For this review, take the finished solid that the model builds, in its own axes (mm). A direction names the side the tool comes from. Coordinates: 2 decimals unless noted, no trailing zeros. Loops run counter-clockwise (first coordinate to the right, second up) from the corner with the lowest first, then second, coordinate; pieces in that order, holes last. Notation, with made-up numbers: (-5.75, 58) - (52.25, 58) arc R22 ccw to (52.25, 88) - close; hole circle Ø5 at (-26.5, 85.25). An arc over 180 degrees is marked (long way). One line per item, written item: value. Start each with the question number.
1. Take a section at D-D, the plane y = -0.3. Count the separate pieces of the cut face and the enclosed holes in it, and give its area (3 significant figures).
2. The part is to be moulded in two halves that separate along Z. For faces 1 (the face through (-1.356, 1, -6)), 2 (the face through (0.739, 0.144, -15.866)), 3 (the face through (0.67, 0.27, -6.81)), say which applies: released by +Z, released by -Z, zero draft, split by the parting line, or undercut.
3. To check wall thickness, follow line 1 (Z direction, x = 1, y = 0.2); line 2 (X direction, y = 1.2, z = -15); line 3 (Z direction, x = 0.6, y = -0.75). State the ranges of each line that lie inside material, in increasing order. Write a range as from..to.
4. Take a section at C-C, the plane x = -1.05. State the section outline as (y, z) points.
5. Take a section at A-A, the plane x = 0.55. State the section outline as (y, z) points, and give its area (3 significant figures).
6. Insertion check: pin 1 (1.5 mm diameter, centred on x = -0.5, y = -0.5, fed in from +Z); pin 2 (1.5 mm diameter, centred on x = 0.5, z = -13.5, fed in from -Y) (3 decimals). Each pin has a flat end and moves straight along its axis. Give the tip position at first contact, or say it passes through.
7. For faces 4 (the face through (0.069, -1, -7)), 5 (the face through (0.739, 0.144, -17.695)), list the 3-axis set-ups (+Z, -Z, +X, -X, +Y, -Y) from which the entire face can be reached by the end or side of a thin tool; tool diameter is ignored.
8. Take a section at B-B, the plane z = -11.5. State the section outline as (x, y) points.
```python
from build123d import *

# Parameters (mm, degrees)
BOSS_EXTRUDE1_DEPTH = 2.9972
CUT_EXTRUDE1_DEPTH  = 1.524
SKETCH6_R           = 1.1176
CUT_EXTRUDE3_DEPTH  = 29.630171982
CUT_EXTRUDE4_DEPTH  = 7.62
BOSS_EXTRUDE2_START = 0.4064
SKETCH9_R           = 1.1176
BOSS_EXTRUDE2_DEPTH = 0.4064
SKETCH10_R          = 1.1176
SKETCH10_R_2        = 0.8001
BOSS_EXTRUDE3_DEPTH = 1.8796
SKETCH11_R          = 4.5466
BOSS_EXTRUDE4_DEPTH = 2.54
SKETCH12_R          = 2.8702
CUT_EXTRUDE5_DEPTH  = 2.3749
SKETCH13_R          = 1.524
CUT_EXTRUDE6_DEPTH  = 28.807597626
SKETCH14_R          = 0.8001
CUT_EXTRUDE7_DEPTH  = 29.056286281
CHAMFER1_SIZE       = 0.127
CHAMFER2_SIZE       = 0.127
CHAMFER3_SIZE       = 0.127
SCALE1_SCALE        = 0.6


with BuildPart() as part:
    # Sketch1 → Boss-Extrude1 (new body)
    with BuildSketch(Plane(origin=(0, 0, 0), x_dir=(0, 0, -1), z_dir=(1, 0, 0))):
        with BuildLine():
            Line((24.769539012, 3.626266444), (5.771274976, 5.288399174))
            ThreePointArc((5.771274976, 5.288399174), (0, 0), (5.771274976, -5.288399174))
            Line((5.771274976, -5.288399174), (24.769539012, -3.626266444))
            ThreePointArc((24.769539012, -3.626266444), (28.0924, 0), (24.769539012, 3.626266444))
        make_face()
    extrude(amount=BOSS_EXTRUDE1_DEPTH)

    # Sketch4 → Cut-Extrude1 (cut)
    with BuildSketch(Plane(origin=(2.9972, 0, 0), x_dir=(0, 0, -1), z_dir=(1, 0, 0))):
        with BuildLine():
            Line((24.703126336, 2.867166085), (5.7048623, 4.529298814))
            ThreePointArc((5.7048623, 4.529298814), (0.762, 0), (5.7048623, -4.529298814))
            Line((5.7048623, -4.529298814), (24.703126336, -2.867166085))
            ThreePointArc((24.703126336, -2.867166085), (27.3304, 0), (24.703126336, 2.867166085))
        make_face()
    extrude(amount=-CUT_EXTRUDE1_DEPTH, mode=Mode.SUBTRACT)

    # Sketch6 → Cut-Extrude3 (cut, through all)
    with BuildSketch(Plane(origin=(1.4732, 0, 0), x_dir=(0, 0, -1), z_dir=(1, 0, 0))):
        with Locations((21.2344, 0)):
            Circle(SKETCH6_R)
    extrude(amount=-CUT_EXTRUDE3_DEPTH, mode=Mode.SUBTRACT)

    # Sketch7 → Cut-Extrude4 (cut)
    with BuildSketch(Plane(origin=(2.9972, 0, 0), x_dir=(0, 0, -1), z_dir=(1, 0, 0))):
        with BuildLine():
            Line((5.771274976, -5.288399174), (24.769539012, -3.626266444))
            ThreePointArc((24.769539012, -3.626266444), (28.0924, 0), (24.769539012, 3.626266444))
            Line((24.769539012, 3.626266444), (5.771274976, 5.288399174))
            ThreePointArc((5.771274976, 5.288399174), (0, 0), (5.771274976, -5.288399174))
        make_face()
        with BuildLine():
            Line((24.703126336, 2.867166085), (5.7048623, 4.529298814))
            ThreePointArc((5.7048623, 4.529298814), (0.762, 0), (5.7048623, -4.529298814))
            Line((5.7048623, -4.529298814), (24.703126336, -2.867166085))
            ThreePointArc((24.703126336, -2.867166085), (27.3304, 0), (24.703126336, 2.867166085))
        make_face(mode=Mode.SUBTRACT)
    extrude(amount=-CUT_EXTRUDE4_DEPTH, mode=Mode.SUBTRACT)

    # Sketch9 → Boss-Extrude2 (add)
    with BuildSketch(Plane(origin=(1.4732, 0, 0), x_dir=(0, 0, -1), z_dir=(1, 0, 0)).offset(BOSS_EXTRUDE2_START)):
        with BuildLine():
            Line((24.703126336, 2.867166085), (5.7048623, 4.529298814))
            ThreePointArc((5.7048623, 4.529298814), (0.762, 0), (5.7048623, -4.529298814))
            Line((5.7048623, -4.529298814), (24.703126336, -2.867166085))
            ThreePointArc((24.703126336, -2.867166085), (27.3304, 0), (24.703126336, 2.867166085))
        make_face()
        with Locations((21.2344, 0)):
            Circle(SKETCH9_R, mode=Mode.SUBTRACT)
    extrude(amount=-BOSS_EXTRUDE2_DEPTH)

    # Sketch10 → Boss-Extrude3 (add)
    with BuildSketch(Plane(origin=(1.8796, 0, 0), x_dir=(0, 0, -1), z_dir=(1, 0, 0))):
        with Locations((21.2344, 0)):
            Circle(SKETCH10_R)
        with Locations((21.2344, 0)):
            Circle(SKETCH10_R_2, mode=Mode.SUBTRACT)
    extrude(amount=-BOSS_EXTRUDE3_DEPTH)

    # Sketch11 → Boss-Extrude4 (add)
    with BuildSketch(Plane.ZY):
        with Locations(Location((-5.3086, 0, 0), (0, 0, 95))):
            Circle(SKETCH11_R)
    extrude(amount=BOSS_EXTRUDE4_DEPTH)

    # Sketch12 → Cut-Extrude5 (cut)
    with BuildSketch(Plane.ZY.offset(2.54)):
        with Locations((-5.3086, 0)):
            Circle(SKETCH12_R)
    extrude(amount=-CUT_EXTRUDE5_DEPTH, mode=Mode.SUBTRACT)

    # Sketch13 → Cut-Extrude6 (cut, through all)
    with BuildSketch(Plane.ZY.offset(0.1651)):
        with Locations((-5.3086, 0)):
            Circle(SKETCH13_R)
    extrude(amount=-CUT_EXTRUDE6_DEPTH, mode=Mode.SUBTRACT)

    # Sketch14 → Cut-Extrude7 (cut, through all)
    with BuildSketch(Plane(origin=(1.8796, 0, 0), x_dir=(0, 0, -1), z_dir=(1, 0, 0))):
        with Locations((18.1864, 0)):
            Circle(SKETCH14_R)
        with Locations((15.1384, 0)):
            Circle(SKETCH14_R)
        with Locations((24.2824, 0)):
            Circle(SKETCH14_R)
    extrude(amount=-CUT_EXTRUDE7_DEPTH, mode=Mode.SUBTRACT)

    # Chamfer1
    chamfer1_edges = [part.edges().sort_by_distance(p)[0] for p in [
        (-2.54, -4.529298814, -4.9123377),
        (-2.54, 0, -8.1788),
        (1.8796, 0, -6.8326),
        (-0.1651, 0, -6.8326),
    ]]
    chamfer(chamfer1_edges, length=CHAMFER1_SIZE)

    # Chamfer2
    chamfer2_edges = [part.edges().sort_by_distance(p)[0] for p in [
        (0, 0, -17.3863),
        (1.8796, 0, -17.3863),
        (0, 0, -14.3383),
        (1.8796, 0, -14.3383),
        (0, 0, -23.4823),
        (1.8796, 0, -23.4823),
        (1.8796, 0, -27.3304),
        (1.8796, 3.698232449, -15.203994318),
        (1.8796, 0, -0.762),
        (1.8796, -3.698232449, -15.203994318),
        (0, 0, -20.4343),
        (1.8796, 0, -20.4343),
    ]]
    chamfer(chamfer2_edges, length=CHAMFER2_SIZE)

    # Chamfer3
    # the kernel refuses this chamfer: 0.127 mm, written as the material it takes off along each edge
    with BuildSketch(Plane(origin=(0, -4.557764206, -5.379501386), x_dir=(0.9996219169112968, -0.027391246498850615, -0.002396423548493402), z_dir=(0, 0.08715574274765155, -0.9961946980917461))) as chamfer3_piece_1_section:
        Polygon((CHAMFER3_SIZE * 0.999621916911, -CHAMFER3_SIZE * 0.0274958766106), (-CHAMFER3_SIZE * 0.0274958766106, -CHAMFER3_SIZE * 0.999621916911), (0, 0), align=None)
    chamfer3_piece_1 = extrude(amount=19.397438057, mode=Mode.PRIVATE)
    chamfer3_piece_1 = chamfer3_piece_1 - Plane(origin=(0.042171089, 0, -5.3086), x_dir=(0, 0.9961946980917455, -0.08715574274765824), z_dir=(1, 0, 0)) * Cylinder(4.5466, 40, mode=Mode.PRIVATE)
    add(chamfer3_piece_1, mode=Mode.SUBTRACT)
    with BuildSketch(Plane(origin=(0, 2.867166085, -24.703126336), x_dir=(-0.027495876610586393, -0.9958180537233419, 0.08712279063523509), z_dir=(0, 0.08715574274765134, 0.9961946980917462))) as chamfer3_piece_2_section:
        Polygon((CHAMFER3_SIZE * 0.999621916911, CHAMFER3_SIZE * 0.0274958766106), (-CHAMFER3_SIZE * 0.0274958766106, CHAMFER3_SIZE * 0.999621916911), (0, 0), align=None)
    chamfer3_piece_2 = extrude(amount=19.397438057, mode=Mode.PRIVATE)
    chamfer3_piece_2 = chamfer3_piece_2 - Plane(origin=(0.042171094, 0, -5.3086), x_dir=(0, 0.9961946980917455, -0.08715574274765824), z_dir=(1, 0, 0)) * Cylinder(4.5466, 40, mode=Mode.PRIVATE)
    add(chamfer3_piece_2, mode=Mode.SUBTRACT)
    with BuildSketch(Plane(origin=(0, 0, -24.452281807), x_dir=(0, -0.996194698091746, -0.08715574274765267), z_dir=(0, -0.08715574274765267, 0.996194698091746))) as chamfer3_piece_3:
        Polygon((2.878118193 - CHAMFER3_SIZE, 0), (2.878118193, CHAMFER3_SIZE), (2.878118193, 0), align=None)
    revolve(axis=Axis((0, 0, -24.452281807), (1, 0, 0)), revolution_arc=170, mode=Mode.SUBTRACT)


with BuildPart() as part_1:
    # Scale1: scaled about (0.419801812, 0, -11.241664116)
    add(part.part.scale(SCALE1_SCALE).moved(Location((0.167920725, 0, -4.496665646))))


solid = part_1.part
```
Solutions:
1. separate pieces: 6
1. enclosed holes: 0
1. area: 15.8 mm2
2. face 1: zero draft
2. face 2: undercut
2. face 3: undercut
3. line 1: -20.88..-19.5, -18.63..-17.67, -16.8..-15.84, -14.97..-14.02, -13.14..-8.57, -6.79..-4.96
3. line 2: 0.17..1.3
3. line 3: -20.72..-8.2, -7.16..-5.06
4. outline: circle Ø5.46 at (0, -7.68); hole circle Ø3.44 at (0, -7.68)
5. outline: (-2.72, -7.92) - (-1.72, -19.32) arc R1.73 ccw to (1.72, -19.32) - (2.72, -7.92) arc R2.73 ccw (long way) to start; hole circle Ø1.83 at (0, -7.68); hole circle Ø0.96 at (0, -19.07); hole circle Ø0.96 at (0, -17.24); hole circle Ø0.96 at (0, -15.41); hole circle Ø0.96 at (0, -13.58)
5. area: 62.2 mm2
6. pin 1: z = -4.95
6. pin 2: y = -2.295
7. face 4: -X
7. face 5: +X, -X
8. outline: (0.17, -2.33) - (0.24, -2.4) - (1.22, -2.4) - (1.3, -2.33) - (1.3, 2.33) - (1.22, 2.4) - (0.24, 2.4) - (0.17, 2.33) - close
